Verification items for the finished model (mm, model axes). A direction names the side the tool comes from. Give positions to 0.01 mm unless a question says otherwise; leave off trailing zeros. Order: outer loops, then holes, each group sorted by start corner. A loop starts at its lowest first (then second) coordinate and runs counter-clockwise, first axis right, second up. Notation, with made-up numbers: (19.5, -19) -> (57.5, -19) arc R19 ccw to (57.5, 12) -> close; hole circle Ø1 at (33, -22.5). An arc over 180 degrees is marked (long way). One line per question, with ' | ' between items. Start each with the question number.
Q1. Access from +Z, -Z, +X, -X, +Y, -Y to the whole of each face (thin tool, end or side, straight path). Record for faces 1 (the cylindrical face through (2.6, 2.5, 8.3)), 2 (the cylindrical face through (-4.06, 22.786, 9.367)), 3 (the flat face through (13, 12, 9)).
Q2. Section check A-A on z = 9.5. Record the cut outline in (x, y), plus the area to 3 significant figures.
Q3. Section check D-D on x = 3.5. Record the cut outline in (y, z).
Q4. Go/stop test with flat-tipped pins: pin 1 (2.5 mm diameter, centred on x = 16.5, z = 9.5, fed in from +Y); pin 2 (3 mm diameter, centred on x = -6.5, z = 3.5, fed in from -Y); pin 3 (4 mm diameter, centred on x = -0.5, z = 8, fed in from +Y). Record where each tip stops, or that it passes through.
Q5. Section check C-C on y = 28.5. Record the cut outline in (x, z).
Q6. Mould release check, pull along Z, two halves, no side actions. Record for faces 4 (the flat face through (17, 5, 7)), 5 (the flat face through (10, 24, 19)), 6 (the flat face through (10, 29, 2)): released by +Z, released by -Z, zero draft, split by the parting line, or undercut.
Q7. Section check B-B on z = 5.5. Record the cut outline in (x, y), plus the area to 3 significant figures.
Q8. Material ranges on probe 1 along Z at (x, y) = (11, 28); probe 2 along Z at (x, y) = (16.5, 2.8); probe 3 along X at (y, z) = (2, 2.5), recorded low to high. Write a range as [from, to].
from build123d import *

# Parameters (mm, degrees)
BOSS_EXTRUDE1_DEPTH = 19
BOSS_EXTRUDE2_REACH = 52.283
SKETCH2_W           = 45
SKETCH2_H           = 2
SKETCH3_R           = 1.5
CUT_EXTRUDE1_DEPTH  = 5


with BuildPart() as part:
    # Sketch1 → Boss-Extrude1 (new body)
    with BuildSketch(Plane.XY):
        with BuildLine():
            Line((0, 5), (0, 0))
            Line((0, 0), (20, 0))
            Line((20, 0), (20, 5))
            Line((20, 5), (13, 5))
            Line((13, 5), (13, 19.161178186))
            ThreePointArc((13, 19.161178186), (23.920180244, 22.705379567), (32.5, 30.334166688))
            Line((32.5, 30.334166688), (32.5, 33.334166688))
            ThreePointArc((32.5, 33.334166688), (10, 22), (-12.5, 33.334166688))
            Line((-12.5, 33.334166688), (-12.5, 30.334166688))
            ThreePointArc((-12.5, 30.334166688), (-3.920180244, 22.705379567), (7, 19.161178186))
            Line((7, 19.161178186), (7, 5))
            Line((7, 5), (0, 5))
        make_face()
    extrude(amount=BOSS_EXTRUDE1_DEPTH)

    # Sketch2 → Boss-Extrude2 (add, up to next)
    with BuildSketch(Plane(origin=(0, 33.334166688, 0), x_dir=(1, 0, 0), z_dir=(0, 1, 0)), mode=Mode.PRIVATE) as boss_extrude2_sk1:
        with Locations((10, -18)):
            Rectangle(SKETCH2_W, SKETCH2_H)
    boss_extrude2_tool1 = extrude(boss_extrude2_sk1.sketch, amount=-BOSS_EXTRUDE2_REACH, mode=Mode.PRIVATE) - part.part
    # Sketch2 → Boss-Extrude2 (add, up to next)
    with BuildSketch(Plane(origin=(0, 33.334166688, 0), x_dir=(1, 0, 0), z_dir=(0, 1, 0)), mode=Mode.PRIVATE) as boss_extrude2_sk2:
        with Locations((10, -1)):
            Rectangle(SKETCH2_W, SKETCH2_H)
    boss_extrude2_tool2 = extrude(boss_extrude2_sk2.sketch, amount=-BOSS_EXTRUDE2_REACH, mode=Mode.PRIVATE) - part.part
    add(boss_extrude2_tool1.solids().sort_by_distance((10, 33.334167, 18))[0])
    add(boss_extrude2_tool2.solids().sort_by_distance((10, 33.334167, 1))[0])

    # Sketch3 → Cut-Extrude1 (cut)
    with BuildSketch(Plane(origin=(0, 5, 0), x_dir=(1, 0, 0), z_dir=(0, 1, 0))):
        with Locations(Location((16.5, -9.5, 0), (0, 0, 180))):
            Circle(SKETCH3_R)
        with Locations(Location((3.5, -9.5, 0), (0, 0, 270))):
            Circle(SKETCH3_R)
    extrude(amount=-CUT_EXTRUDE1_DEPTH, mode=Mode.SUBTRACT)


solid = part.part
Filled in:
1) face 1: -Y | face 2: +Z, -Z, -X | face 3: +Z, -Z, +X
2) outline: (-12.5, 30.33) arc R28 ccw to (7, 19.16) -> (7, 5) -> (5, 5) -> (5, 0) -> (15, 0) -> (15, 5) -> (13, 5) -> (13, 19.16) arc R28 ccw to (32.5, 30.33) -> (32.5, 33.33) arc R28 cw to (-12.5, 33.33) -> close; (0, 0) -> (2, 0) -> (2, 5) -> (0, 5) -> close; (18, 0) -> (20, 0) -> (20, 5) -> (18, 5) -> close | area: 289 mm²
3) outline: (0, 0) -> (5, 0) -> (5, 8) -> (0, 8) -> close; (0, 11) -> (5, 11) -> (5, 19) -> (0, 19) -> close; (19.76, 0) -> (33.33, 0) -> (33.33, 2) -> (22.76, 2) -> (22.76, 17) -> (33.33, 17) -> (33.33, 19) -> (19.76, 19) -> close
4) pin 1: y = 23.09 | pin 2: y = 23.36 | pin 3: y = 24.95
5) outline: (-11.02, 0) -> (31.02, 0) -> (31.02, 19) -> (-11.02, 19) -> close; hole (-7.94, 2) -> (27.94, 2) -> (27.94, 17) -> (-7.94, 17) -> close
6) face 4: zero draft | face 5: released by +Z | face 6: undercut
7) outline: (-12.5, 30.33) arc R28 ccw to (7, 19.16) -> (7, 5) -> (0, 5) -> (0, 0) -> (20, 0) -> (20, 5) -> (13, 5) -> (13, 19.16) arc R28 ccw to (32.5, 30.33) -> (32.5, 33.33) arc R28 cw to (-12.5, 33.33) -> close | area: 319 mm²
8) probe 1: [0, 2], [17, 19] | probe 2: [0, 8], [11, 19] | probe 3: [0, 20]
